For this review, use the dimensioned drawing (mm, ordinates from the lowest corner) and the shaded views. A direction names the side the tool comes from. Round coordinates to 2 decimals unless told otherwise and drop trailing zeros. Order: outer loops, then holes, each group sorted by start corner. A loop starts at its lowest first (then second) coordinate and runs counter-clockwise, first axis right, second up. Notation, with made-up numbers: M 53.5,20.25 L 59.5,20.25 A15 ccw 59.5,33.25 Z; hole C 24,-31 d1. An arc over 180 degrees is marked long. Put each result on its own line as item: value.
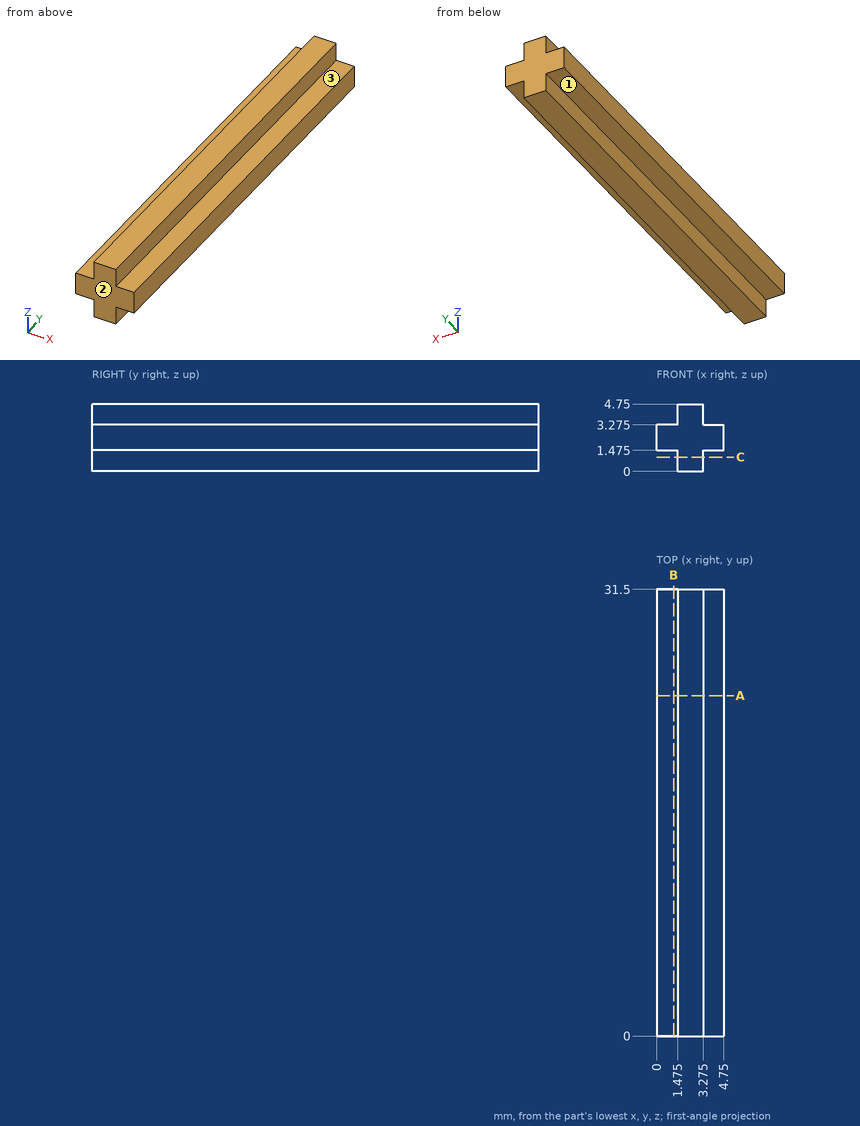
(1) Add section A-A on y = 24. Give the boundary of the cut face in (x, z) (3 decimals).
A:
outline: M 0,1.475 L 1.475,1.475 L 1.475,0 L 3.275,0 L 3.275,1.475 L 4.75,1.475 L 4.75,3.275 L 3.275,3.275 L 3.275,4.75 L 1.475,4.75 L 1.475,3.275 L 0,3.275 Z
(2) To check wall thickness, follow L1, parallel to Z at x = 1.1, y = 27 (3 decimals). State the ranges of the line that lie inside material, in increasing order.
A:
L1: z = 1.475 to 3.275
(3) Add section C-C on z = 1. Give the boundary of the cut face in (x, y) (3 decimals).
A:
outline: M 1.475,0 L 3.275,0 L 3.275,31.5 L 1.475,31.5 Z
(4) Insertion check: pin 1 Ø1.2 at (x, y) = (4, 14.5) entering from -Z (3 decimals); pin 2 Ø0.7 at (y, z) = (15, 4) entering from +X (3 decimals); pin 3 Ø1.6 at (y, z) = (22.5, 1) entering from +X; pin 4 Ø0.7 at (y, z) = (20.5, 4.5) entering from -X (3 decimals). Each pin has a flat end and moves straight along its axis. Give the tip position at first contact, or say it passes through.
A:
pin 1: stops at z = 1.475
pin 2: stops at x = 3.275
pin 3: stops at x = 4.75
pin 4: stops at x = 1.475
(5) For the marked faces 1, 2 and 3, list the 3-axis set-ups (+Z, -Z, +X, -X, +Y, -Y) from which the entire face can be reached by the end or side of a thin tool; tool diameter is ignored.
A:
face 1: -Z, -X, +Y, -Y
face 2: +Z, -Z, +X, -X, -Y
face 3: +Z, +X, +Y, -Y
(6) Add section B-B on x = 1.2. Give the boundary of the cut face in (y, z) (3 decimals), then the cut area to 3 significant figures.
A:
outline: M 0,1.475 L 31.5,1.475 L 31.5,3.275 L 0,3.275 Z
area: 56.7 mm2
